CAD build for the part. Positions are in the model's coordinates, mm. Face numbers are marked on the shaded views. Give positions to 0.01 mm unless a question says otherwise; leave off trailing zeros. Order: outer loops, then holes, each group sorted by start corner. A loop starts at its lowest first (then second) coordinate and runs counter-clockwise, first axis right, second up.
Item 1: Band-saw the part on C-C on z = -3. Give the cut face in (x, y).
Item 2: Two-plate mould, pull along Z, no slides. Class the marked faces 1, 2 and 3: released by +Z, released by -Z, zero draft, split by the parting line, or undercut.
Item 3: Band-saw the part on D-D on y = -45.5. Give the cut face in (x, z), plus the area to 3 significant figures.
Item 4: Band-saw the part on A-A on y = -75. Give the cut face in (x, z), plus the area to 3 significant figures.
Item 5: Band-saw the part on B-B on x = -2. Give the cut face in (y, z), plus the area to 3 significant figures.
Item 6: Flat gauge pins, fed straight in: P1, Ø6, axis at y = -57, z = 19.5, coming from the -X side; P2, Ø10, axis at y = -42, z = 23, coming from the +X side; P3, Ø10, axis at x = 18.5, y = -32, coming from the +Z side. Where does each tip first touch, or does it go through?
Item 7: Wall check: L1, parallel to X at y = -48.5, z = 7; L2, parallel to Z at x = 0, y = -22; L3, parallel to Z at x = 5, y = -56. Give the ranges that are in metal, low to high.
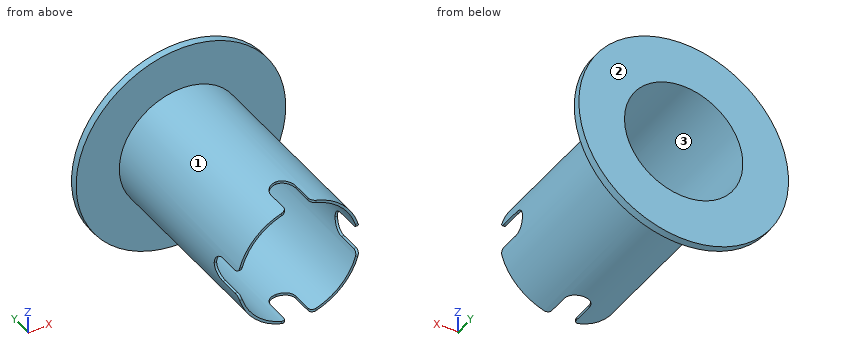
```python
from build123d import *

# Parameters (mm, degrees)
F0_R     = 42.5
F0_R_2   = 25
F1_DEPTH = 3
F0_R_3   = 24
F3_DEPTH = 80
F5_DEPTH = 2
F6_COUNT = 4
F7_R     = 2


with BuildPart() as f1:
    # F0 (on Front) → F1 (new body)
    with BuildSketch(Plane.XZ):
        Circle(F0_R)
        Circle(F0_R_2, mode=Mode.SUBTRACT)
    extrude(amount=F1_DEPTH)

    # F0 (on Front) → F3 (join)
    with BuildSketch(Plane.XZ):
        Circle(F0_R_2)
        Circle(F0_R_3, mode=Mode.SUBTRACT)
    extrude(amount=F3_DEPTH)

    # F6: F5 ×4 about axis
    f6_axis = Axis((0, -80, 0), (0, -1, 0))


with BuildPart() as f5:
    # F4 (on offset) → F5 (new body)
    with BuildSketch(Plane.XY.offset(25)):
        with BuildLine():
            Line((-5, -70), (-5, -80))
            Line((-5, -80), (5, -80))
            Line((5, -80), (5, -70))
            ThreePointArc((5, -70), (3.5355339059, -66.4644660941), (0, -65))
            ThreePointArc((0, -65), (-3.5355339059, -66.4644660941), (-5, -70))
        make_face()
    extrude(amount=-F5_DEPTH)


with BuildPart() as f1_1:
    add(f1.part)
    for i in range(1, F6_COUNT):
        add(f5.part.rotate(f6_axis, i * 360 / F6_COUNT), mode=Mode.SUBTRACT)

    # F6#seed: cut F5
    add(f5.part, mode=Mode.SUBTRACT)

    # F7
    f7_edges = [f1_1.edges().sort_by_distance(p)[0] for p in [
        (5, -80, -23.984143),
        (-5, -80, -23.984143),
        (23.984143, -80, -5),
        (23.984143, -80, 5),
        (5, -80, 23.984143),
        (-5, -80, 23.984143),
        (-23.984143, -80, -5),
        (-23.984143, -80, 5),
    ]]
    fillet(f7_edges, radius=F7_R)


solid = f1_1.part
```
The answers:
1. outline: (-42.39, -3) - (-24.82, -3) - (-24.82, -66) - (-23.81, -66) - (-23.81, 0) - (-42.39, 0) - close; (23.81, -66) - (24.82, -66) - (24.82, -3) - (42.39, -3) - (42.39, 0) - (23.81, 0) - close
2. face 1: split by the parting line
2. face 2: zero draft
2. face 3: undercut
3. outline: circle Ø50 at (0, 0); hole circle Ø48 at (0, 0)
3. area: 154 mm2
4. outline: (-24.49, -5) arc R25 ccw to (-5, -24.49) - (-5, -23.47) arc R24 cw to (-23.47, -5) - close; (-24.49, 5) - (-23.47, 5) arc R24 cw to (-5, 23.47) - (-5, 24.49) arc R25 ccw to start; (5, -24.49) arc R25 ccw to (24.49, -5) - (23.47, -5) arc R24 cw to (5, -23.47) - close; (5, 23.47) arc R24 cw to (23.47, 5) - (24.49, 5) arc R25 ccw to (5, 24.49) - close
4. area: 114 mm2
5. outline: (-65.42, -24.92) - (-3, -24.92) - (-3, -42.45) - (0, -42.45) - (0, -23.92) - (-65.42, -23.92) - close; (-65.42, 23.92) - (0, 23.92) - (0, 42.45) - (-3, 42.45) - (-3, 24.92) - (-65.42, 24.92) - close
5. area: 236 mm2
6. P1: stops at x = -18.78
6. P2: stops at x = 17.35
6. P3: stops at z = 21.04
7. L1: x = -24 to -22.96, 22.96 to 24
7. L2: z = -25 to -24, 24 to 25
7. L3: z = -24.49 to -23.47, 23.47 to 24.49
